from build123d import *

# Parameters (mm, degrees)
F1_DEPTH = 3
F4_R     = 2
F5_DEPTH = 2


with BuildPart() as f1:
    # F0 (on Top) → F1 (new body)
    with BuildSketch(Plane.XY):
        Polygon((2.020726, -3.5), (4.041452, 0), (2.020726, 3.5), (-2.020726, 3.5), (-4.041452, 0), (-2.020726, -3.5), align=None)
    extrude(amount=F1_DEPTH)

    # F2 (on Right) → F3 (revolve)
    with BuildSketch(Plane.YZ):
        Polygon((-0.4, 4.75), (-2, 3), (-0.2, 3), (-0.2, 4.75), align=None)
    revolve(axis=Axis((0, 0, 3.308563), (0, 0, 1)))

    # F4 (on face) → F5 (cut)
    with BuildSketch(Plane(origin=(0, 0, 0), x_dir=(1, 0, 0), z_dir=(0, 0, -1))):
        Circle(F4_R)
    extrude(amount=-F5_DEPTH, mode=Mode.SUBTRACT)


solid = f1.part
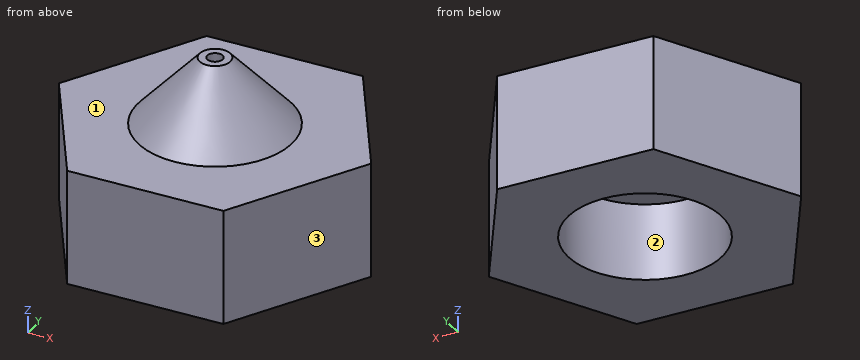
Work out the finished part from the listing and answer in its coordinate system (mm). Face numbers are marked on the shaded views. Give positions to 0.01 mm unless a question says otherwise; leave off trailing zeros. Order: outer loops, then holes, each group sorted by start corner. A loop starts at its lowest first (then second) coordinate and runs counter-clockwise, first axis right, second up. Notation, with made-up numbers: (-22, 9.5) -> (35, 9.5) arc R18 cw to (35, 41.5) -> close; hole circle Ø6 at (86.25, 38). An arc over 180 degrees is marked (long way). Answer as a JSON object with one key per item and string values. Group by question number.
1. Section C-C on z = 4.4 is taken. Determine the outline of the cut face in (x, y).
2. Section B-B on x = 0 is taken. Determine the outline of the cut face in (y, z).
3. Consider line 1 along Y through (x, z) = (0, 1.4); line 2 along Z through (x, y) = (-0.25, 0); line 3 along X through (y, z) = (0.5, 1). Determine where each line is inside the solid, lowest interval first. Write a range as [from, to].
4. Section A-A on z = 1.55 is taken. Determine the outline of the cut face in (x, y).
5. Section D-D on x = -2.25 is taken. Determine the outline of the cut face in (y, z).
6. Flat-ended cylindrical pins translate along their axes: pin 1 Ø1.5 at (y, z) = (-1.5, 0.5) entering from -X; pin 2 Ø1.2 at (x, y) = (-0.5, -1) entering from -Z; pin 3 Ø1.5 at (x, y) = (-3, 3) entering from +Z. Find the tip coordinate at first contact, or state that the pin passes through.
7. The mould has two halves that part along X. Classify the marked faces 1, 2 and 3: released by +X, released by -X, zero draft, split by the parting line, or undercut.
Result sheet:
{
 "1": {"outline": "circle Ø1.44 at (0, 0); hole circle Ø0.4 at (0, 0)"},
 "2": {"outline": "(-3.5, 0) -> (-2, 0) -> (-2, 2) -> (2, 2) -> (2, 0) -> (3.5, 0) -> (3.5, 3) -> (2, 3) -> (0.4, 4.75) -> (0.2, 4.75) -> (0.2, 3) -> (-0.2, 3) -> (-0.2, 4.75) -> (-0.4, 4.75) -> (-2, 3) -> (-3.5, 3) -> close"},
 "3": {"line 1": "y = [-3.5, -2], [2, 3.5]", "line 2": "z = [2, 4.75]", "line 3": "x = [-3.75, -1.94], [1.94, 3.75]"},
 "4": {"outline": "(-4.04, 0) -> (-2.02, -3.5) -> (2.02, -3.5) -> (4.04, 0) -> (2.02, 3.5) -> (-2.02, 3.5) -> close; hole circle Ø4 at (0, 0)"},
 "5": {"outline": "(-3.1, 0) -> (3.1, 0) -> (3.1, 3) -> (-3.1, 3) -> close"},
 "6": {"pin 1": "stops at x = -3.61", "pin 2": "stops at z = 2", "pin 3": "stops at z = 3"},
 "7": {"face 1": "zero draft", "face 2": "undercut", "face 3": "released by +X"}
}
